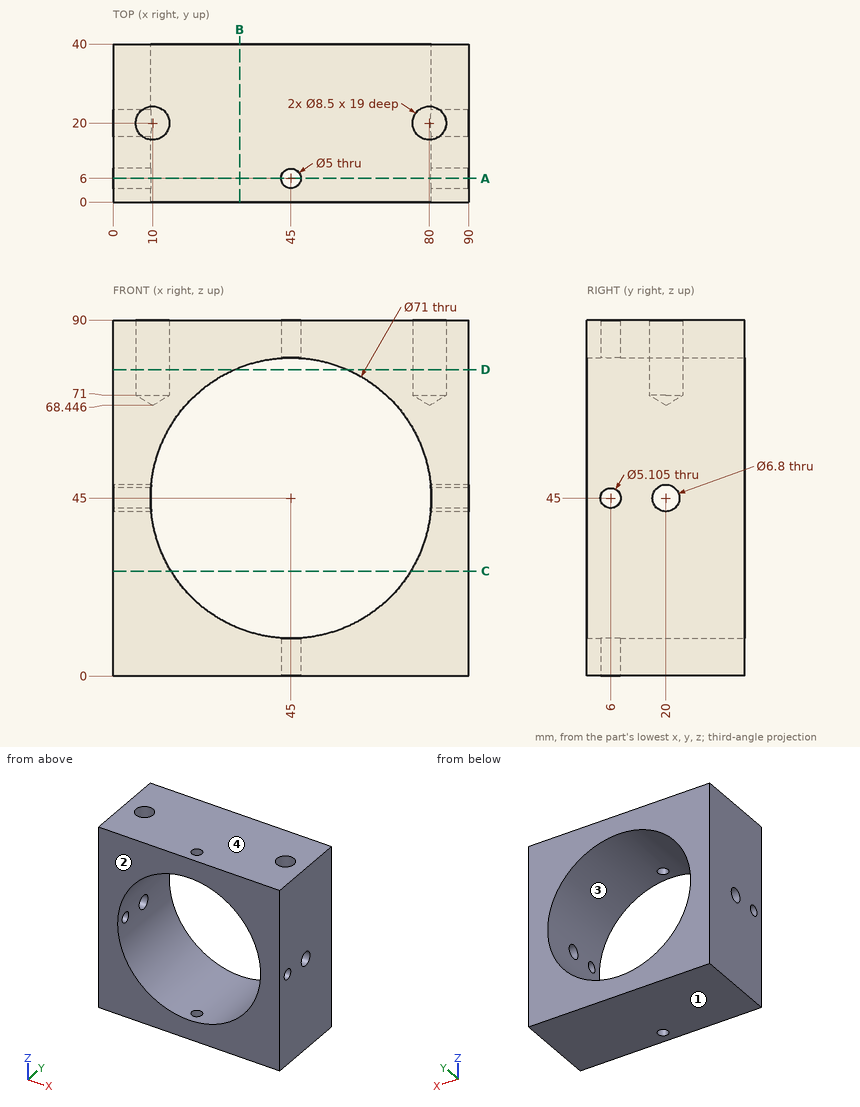
Part print with two shaded views. Sizes in mm from the minimum x, y, z corner. Coordinates: 2 decimals unless noted, no trailing zeros. Order: outer loops, then holes, each group sorted by start corner. A loop starts at its lowest first (then second) coordinate and runs counter-clockwise, first axis right, second up. Notation, with made-up numbers: M 63.25,82.5 L 84.25,82.5 A16 cw 84.25,105.5 Z; hole C 69,79 d5. An arc over 180 degrees is marked long. One line per question, with ' | ' between items. Start each with the question number.
1. Cut at D-D (z = 77.5). Write the cut outline in (x, y).
2. Wall check: line 1 along Z through (x, y) = (44.5, 21.5); line 2 along Y through (x, z) = (45, 4.5); line 3 along Y through (x, z) = (10, 78). Give the ranges that are in metal, low to high. Write a range as [from, to].
3. Mould opens along Z. For the marked faces 1, 2, 3 and 4 say: +Z half, -Z half, draft (parallel to the pull), parting line (faces both ways), or undercut.
4. Cut at B-B (x = 32). Write the cut outline in (y, z), plus the area to 3 significant figures.
5. Cut at A-A (y = 6). Write the cut outline in (x, z), plus the area to 3 significant figures.
6. Cut at C-C (z = 26.5). Write the cut outline in (x, y), plus the area to 3 significant figures.
The answers:
1) outline: M 0,0 L 30.72,0 L 30.72,40 L 0,40 Z; M 59.28,0 L 90,0 L 90,40 L 59.28,40 Z; hole C 10,20 d8.5; hole C 80,20 d8.5
2) line 1: z = [0, 9.5], [80.5, 90] | line 2: y = [0, 3.5], [8.5, 40] | line 3: y = [0, 15.75], [24.25, 40]
3) face 1: -Z half | face 2: draft | face 3: undercut | face 4: +Z half
4) outline: M 0,0 L 40,0 L 40,11.97 L 0,11.97 Z; M 0,78.03 L 40,78.03 L 40,90 L 0,90 Z | area: 957 mm2
5) outline: M 0,0 L 42.5,0 L 42.5,9.59 A35.5 cw 9.59,42.45 L 0,42.45 Z; M 0,47.55 L 9.59,47.55 A35.5 cw 42.5,80.41 L 42.5,90 L 0,90 Z; M 47.5,0 L 90,0 L 90,42.45 L 80.41,42.45 A35.5 cw 47.5,9.59 Z; M 47.5,80.41 A35.5 cw 80.41,47.55 L 90,47.55 L 90,90 L 47.5,90 Z | area: 3,950 mm2
6) outline: M 0,0 L 14.7,0 L 14.7,40 L 0,40 Z; M 75.3,0 L 90,0 L 90,40 L 75.3,40 Z | area: 1,180 mm2
